from build123d import *

# Parameters (mm, degrees)
PAD008_DEPTH        = 2
PAD009_DEPTH        = 1
POCKET009_DEPTH     = 3.001
HOLE006_D           = 4
HOLE006_DEPTH       = 25
HOLE006_CSINK_D     = 9
HOLE006_CSINK_ANGLE = 90
FILLET007_R         = 1


with BuildPart() as part:
    # Sketch025 → Pad008 (new body)
    with BuildSketch(Plane.XZ):
        with BuildLine():
            Line((17, 28), (-17, 28))
            ThreePointArc((-17, 28), (-21.242641, 26.242641), (-23, 22))
            Line((-23, 22), (-23, -30))
            Line((-23, -30), (27, -30))
            Line((27, -30), (27, -18.583005))
            ThreePointArc((23, -8), (24.03337, -13.656854), (27, -18.583005))
            Line((23, 22), (23, -8))
            ThreePointArc((23, 22), (21.242641, 26.242641), (17, 28))
        make_face()
    extrude(amount=-PAD008_DEPTH)

    # Sketch026 (on Face9 of Pad008) → Pad009 (join)
    with BuildSketch(Plane.XZ):
        with BuildLine():
            Line((-20.75, -20.75), (-20.75, 20.75))
            ThreePointArc((-15.75, 25.75), (-19.285534, 24.285534), (-20.75, 20.75))
            Line((-15.75, 25.75), (15.75, 25.75))
            ThreePointArc((20.75, 20.75), (19.285534, 24.285534), (15.75, 25.75))
            Line((20.75, 20.75), (20.75, -15.935045))
            Line((20.75, -15.935045), (25, -23.296261))
            Line((25, -23.296261), (20.75, -25.75))
            Line((20.75, -25.75), (-15.75, -25.75))
            ThreePointArc((-20.75, -20.75), (-19.285534, -24.285534), (-15.75, -25.75))
        make_face()
    extrude(amount=PAD009_DEPTH)

    # Sketch027 (on Face5 of Pad009) → Pocket009 (cut, through all)
    with BuildSketch(Plane(origin=(0, 2, 0), x_dir=(1, 0, 0), z_dir=(0, 1, 0))):
        with BuildLine():
            Line((-6, -28), (6, -28))
            Line((6, -28), (3.46582, -10))
            ThreePointArc((3.46582, -10), (0, -6.987945), (-3.46582, -10))
            Line((-6, -28), (-3.46582, -10))
        make_face()
    extrude(amount=-POCKET009_DEPTH, mode=Mode.SUBTRACT)

    # Hole006
    with Locations(Plane(origin=(0, 2, 0), x_dir=(1, 0, 0), z_dir=(0, 1, 0))):
        with Locations((-15, -20), (15, -20), (4, 5)):
            CounterSinkHole(HOLE006_D / 2, HOLE006_CSINK_D / 2, depth=HOLE006_DEPTH, counter_sink_angle=HOLE006_CSINK_ANGLE)

    # Fillet007
    fillet007_edges = [part.edges().sort_by_distance(p)[0] for p in [
        (23, 2, 7),
        (24.03337, 2, -13.656854),
        (27, 2, -24.291503),
        (2, 2, -30),
        (-23, 2, -4),
        (-21.242641, 2, 26.242641),
        (-11.5, 2, 28),
        (-4.73291, 2, 19),
        (0, 2, 6.987945),
        (4.73291, 2, 19),
        (11.5, 2, 28),
        (21.242641, 2, 26.242641),
    ]]
    fillet(fillet007_edges, radius=FILLET007_R)


solid = part.part
The model under review builds one solid part; all positions refer to its coordinate system, in mm. A direction names the side the tool comes from. Round coordinates to 2 decimals unless told otherwise and drop trailing zeros. Loops run counter-clockwise (first coordinate to the right, second up) from the corner with the lowest first, then second, coordinate; pieces in that order, holes last. Notation, with made-up numbers: (62, 17) -> (93, 17) arc R25 ccw to (93, 44) -> close; hole circle Ø2 at (16, 26.25). An arc over 180 degrees is marked (long way). Write item = value, one per line. Start each with the question number.
Item 1: Take a section at C-C on z = 20. Count the separate pieces of the cut face and the enclosed holes in it, plus the area to 3 significant figures.
Item 2: Take a section at A-A on x = 15. Give the boundary of the cut face in (y, z), plus the area to 3 significant figures.
Item 3: Take a section at B-B on z = -5. Give the boundary of the cut face in (x, y).
Item 4: Insertion check: pin 1 (5 mm diameter, centred on x = -11.5, z = 17.5, fed in from +Y); pin 2 (0.8 mm diameter, centred on y = 0.5, z = 3.5, fed in from +X); pin 3 (6.5 mm diameter, centred on x = 4, z = -5, fed in from +Y); pin 4 (0.8 mm diameter, centred on x = -11, y = -0.5, fed in from +Z). Each pin has a flat end and moves straight along its axis. Give the tip position at first contact, or say it passes through.
Item 5: Mouldability with a two-part tool opening along X and no side actions: class faces 6 (the conical face through (16.564, -0.379, 18.566)), 7 (the flat face through (2, 0, -27)), 8 (the flat face through (22.9, -0.49, -24.51)) as released by +X, released by -X, zero draft, split by the parting line, or undercut.
Item 6: To check wall thickness, follow L1, parallel to Z at x = 15, y = -0.75; L2, parallel to X at y = -0.85, z = 20; L3, parallel to X at y = 1.05, z = 21.5. State the ranges of each line that lie inside material, in increasing order.
Item 7: For faces 1 (the cylindrical face through (-5, 1.7, 18.83)), 2 (the cylindrical face through (-19.32, -0.49, -24.25)), 3 (the cylindrical face through (-19.25, -0.49, 24.32)), 4 (the flat face through (4.75, 0.01, 19.13)), 5 (the cylindrical face through (19.32, -0.49, 24.25)), list the 3-axis set-ups (+Z, -Z, +X, -X, +Y, -Y) from which the entire face can be reached by the end or side of a thin tool; tool diameter is ignored.
Result:
q1.separate_pieces = 4
q1.enclosed_holes = 0
q1.area = 66.9 mm²
q2.outline = (-1, -25.75) -> (0, -25.75) -> (0, -30) -> (1, -30) arc R1 ccw to (2, -29) -> (2, 15.5) -> (-0.5, 18) -> (-1, 18) -> close; (-1, 22) -> (-0.5, 22) -> (2, 24.5) -> (2, 27) arc R1 ccw to (1, 28) -> (0, 28) -> (0, 25.75) -> (-1, 25.75) -> close
q2.area = 149 mm²
q3.outline = (-23, 0) -> (-20.75, 0) -> (-20.75, -1) -> (2, -1) -> (2, -0.5) -> (-0.5, 2) -> (-22, 2) arc R1 ccw to (-23, 1) -> close; (6, -1) -> (20.75, -1) -> (20.75, 0) -> (23, 0) -> (23, 1) arc R1 ccw to (22, 2) -> (8.5, 2) -> (6, -0.5) -> close
q4.pin_1 = 2
q4.pin_2 = 23
q4.pin_3 = 0.75
q4.pin_4 = 25.75
q5.face_6 = undercut
q5.face_7 = zero draft
q5.face_8 = released by +X
q6.L1 = -25.75 to 18, 22 to 25.75
q6.L2 = -20.75 to -17, -13 to -4.87, 4.87 to 13, 17 to 20.75
q6.L3 = -23 to -18.22, -11.78 to -5.09, 5.09 to 11.78, 18.22 to 23
q7.face_1 = +Z, +Y
q7.face_2 = -Z, -X, -Y
q7.face_3 = +Z, -X, -Y
q7.face_4 = +Z, +Y, -Y
q7.face_5 = +Z, +X, -Y
